```python
from build123d import *

# Parameters (mm, degrees)
CUT_EXTRUDE1_DEPTH      = 30.212509527
CUT_EXTRUDE1_DEPTH_BACK = 30.212509527
SKETCH2_R               = 5.55625
SKETCH4_R               = 2.15
CUT_EXTRUDE3_DEPTH      = 5
CIRPATTERN1_COUNT       = 6
CUT_EXTRUDE4_REACH      = 45.605
CUT_EXTRUDE4_END_RADIUS = 5.55625
SKETCH6_R               = 5.555


with BuildPart() as part:
    # Sketch1 → Revolve1 (revolve)
    with BuildSketch(Plane.XY, mode=Mode.PRIVATE) as revolve1_sk:
        Polygon((0, -18.690625), (15.875, -18.690625), (15.875, -3.690625), (14.29, -3.690625), (14.29, 8.809375), (12.7, 10.399375), (12.7, 13.809375), (10.31875, 13.809375), (10.31875, 16.190625), (12.7, 16.190625), (12.7, 18.690625), (0, 18.690625), align=None)
    revolve(revolve1_sk.sketch.rotate(Axis((0, -8.095014715, 0), (0, 1, 0)), 90), axis=Axis((0, -8.095014715, 0), (0, 1, 0)))

    # Sketch2 → Cut-Extrude1 (cut, two sides: drawn at the far end of the back side and taken through both)
    with BuildSketch(Plane(origin=(0, 0, 0), x_dir=(0, 0, -1), z_dir=(1, 0, 0)).offset(-CUT_EXTRUDE1_DEPTH_BACK)):
        with Locations((0, -11.190625)):
            Circle(SKETCH2_R)
    extrude(amount=CUT_EXTRUDE1_DEPTH + CUT_EXTRUDE1_DEPTH_BACK, mode=Mode.SUBTRACT)

    # Sketch4 → Cut-Extrude3 (cut)
    with BuildSketch(Plane(origin=(14.29, 0, 0), x_dir=(0, 0, -1), z_dir=(1, 0, 0))):
        with Locations((0, 5.059375)):
            Circle(SKETCH4_R)
    cut_extrude3 = extrude(amount=-CUT_EXTRUDE3_DEPTH, mode=Mode.SUBTRACT)

    # CirPattern1: Cut-Extrude3 ×6 about axis
    cirpattern1_axis = Axis((0, 0, 0), (0, 1, 0))
    for i in range(1, CIRPATTERN1_COUNT):
        add(cut_extrude3.rotate(cirpattern1_axis, i * 360 / CIRPATTERN1_COUNT), mode=Mode.SUBTRACT)

    # Cut-Extrude4: up to this cylinder (the profile starts outside it)
    cut_extrude4_end = Plane(origin=(0, -11.190625, 0), z_dir=(1, 0, 0)) * Cylinder(CUT_EXTRUDE4_END_RADIUS, 103.3225, mode=Mode.PRIVATE)
    # Sketch6 → Cut-Extrude4 (cut, up to the surface)
    with BuildSketch(Plane(origin=(0, 18.690625, 0), x_dir=(1, 0, 0), z_dir=(0, 1, 0)), mode=Mode.PRIVATE) as cut_extrude4_sk1:
        with Locations(Location((0, 0, 0), (0, 0, 270))):
            Circle(SKETCH6_R)
    cut_extrude4_tool1 = extrude(cut_extrude4_sk1.sketch, amount=-CUT_EXTRUDE4_REACH, mode=Mode.PRIVATE) - cut_extrude4_end
    add(cut_extrude4_tool1.solids().sort_by_distance((0, 18.690625, 0))[0], mode=Mode.SUBTRACT)


solid = part.part
```
The listing builds one solid part. Answer for the finished solid, in the listing's coordinates (mm). A direction names the side the tool comes from. Coordinates: 2 decimals unless noted, no trailing zeros. Order: outer loops, then holes, each group sorted by start corner. A loop starts at its lowest first (then second) coordinate and runs counter-clockwise, first axis right, second up. Notation, with made-up numbers: M -38.5,78.5 L -20.5,78.5 A32 cw -20.5,116.5 Z; hole C -2,37 d5. An arc over 180 degrees is marked long. Answer as a JSON object with one key per item and string values. Group by question number.
1. Section A-A on z = 0 is taken. State how many separate pieces and enclosed holes the cut face has, then the cut area to 3 significant figures.
2. Determine the mould class of faces 5 (the cylindrical face through (-4.05, 5.15, -11.31)), 6 (the cylindrical face through (14.08, -11.09, -7.33)), 7 (the flat face through (0, -18.691, 0)) for opening direction X: released by +X, released by -X, zero draft, split by the parting line, or undercut.
3. Section D-D on x = 0 is taken. Write down the section's boundary in (y, z) (1 decimal).
4. Flat-ended cylindrical pins translate along their axes: P1, Ø3, axis at x = -12, y = -11, coming from the +Z side; P2, Ø4.5, axis at y = 4.5, z = -1, coming from the +X side; P3, Ø10, axis at y = -11.19, z = 0, coming from the +X side; P4, Ø5.5, axis at y = 5.06, z = 0, coming from the -X side. Find the tip coordinate at first contact, or state that the pin passes through.
5. Straight lines are drawn through the part: line 1 (Y direction, x = 11, z = 0); line 2 (Y direction, x = 9.5, z = -1.5); line 3 (Y direction, x = 12.8, z = 0). For each, find the intervals that lie inside material, in ascending order.
6. Section C-C on y = 15.5 is taken. Write down the section's boundary in (x, z) (1 decimal).
7. A tool of negligible diameter and unlimited length cuts with its end or side. For faces 1 (the cylindrical face through (7.7, 17.5, 10.1)), 2 (the flat face through (9.29, 5, 0)), 3 (the cylindrical face through (-11.83, 5.15, -2.15)), 4 (the flat face through (-4.62, 5.09, -8.06)), from which of +Z, -Z, +X, -X, +Y, -Y can it reach the whole face along a straight path? Write none if from no direction.
Values follow:
{
 "1": {"separate pieces": "3", "enclosed holes": "0", "area": "410 mm2"},
 "2": {"face 5": "undercut", "face 6": "split by the parting line", "face 7": "zero draft"},
 "3": {"outline": "M -18.7,-15.9 L -3.7,-15.9 L -3.7,-14.3 L 8.8,-14.3 L 10.4,-12.7 L 13.8,-12.7 L 13.8,-10.3 L 16.2,-10.3 L 16.2,-12.7 L 18.7,-12.7 L 18.7,-5.6 L -11.1,-5.6 A5.6 cw long -11.1,5.6 L 18.7,5.6 L 18.7,12.7 L 16.2,12.7 L 16.2,10.3 L 13.8,10.3 L 13.8,12.7 L 10.4,12.7 L 8.8,14.3 L -3.7,14.3 L -3.7,15.9 L -18.7,15.9 Z"},
 "4": {"P1": "z = 11.91", "P2": "x = 14.29", "P3": "through", "P4": "x = -14.29"},
 "5": {"line 1": "-18.69 to -16.75, -5.63 to 2.91, 7.21 to 13.81, 16.19 to 18.69", "line 2": "-18.69 to -16.54, -5.84 to 3.52, 6.6 to 18.69", "line 3": "-18.69 to -16.75, -5.63 to 2.91, 7.21 to 10.3"},
 "6": {"outline": "C 0,0 d20.6; hole C 0,0 d11.1"},
 "7": {"face 1": "+Y", "face 2": "+X", "face 3": "-X", "face 4": "none"}
}
